Here's how the part is built. I have some questions about the finished solid (model axes, mm). Face numbers are marked on the shaded views. Coordinates: 2 decimals unless noted, no trailing zeros. Order: outer loops, then holes, each group sorted by start corner. A loop starts at its lowest first (then second) coordinate and runs counter-clockwise, first axis right, second up. Notation, with made-up numbers: (59, -30.75) - (109, -30.75) arc R24 cw to (109, -8.75) - close; hole circle Ø8 at (54.5, 13.25). An arc over 180 degrees is marked (long way). Answer in a Markdown table with one row per item. Add a question column.
Item 1: I want a section at B-B (x = 6.5). Please give me the cut outline in (y, z).
Item 2: If I drill on line 1 along Y through (x, z) = (12, 5.5); line 2 along Y through (x, z) = (10.75, 2.75); line 3 along X through (y, z) = (27, 6.25), over which ranges is the centre line in solid material (lowest first)? Write a range as from..to.
Item 3: I want a section at A-A (y = 13.5). Please give me the cut outline in (x, z), plus the area to 3 significant figures.
Item 4: I want a section at C-C (z = 5.25). Please give me the cut outline in (x, y).
Item 5: I want a section at D-D (x = 12). Please give me the cut outline in (y, z).
Item 6: Thinking about a two-plate mould opening in Y: for the marked faces 1, 2, 3 and 4, which applies, +Y half, -Y half, draft (parallel to the pull), parting line (faces both ways), or undercut?
Item 7: Will this pin go through, and if not, where does the flat tip stop? pin 1 Ø11.5 at (x, y) = (12, 17.5) entering from -Z.
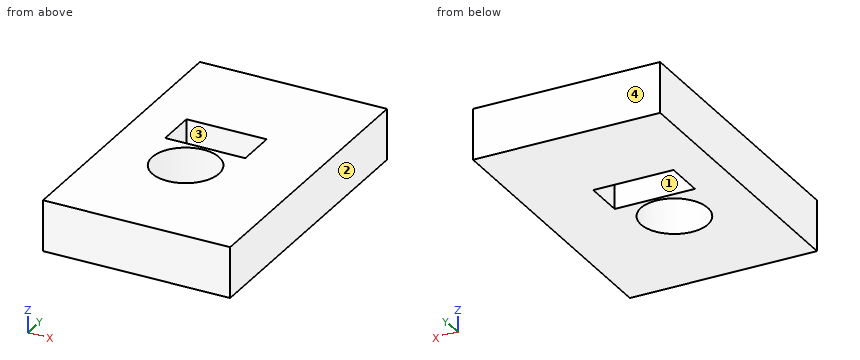
```python
from build123d import *

# Parameters (mm, degrees)
F0_W     = 28
F0_H     = 44
F1_DEPTH = 7.6
F2_R     = 5
F2_W     = 12
F2_H     = 6
F3_DEPTH = 7.601


with BuildPart() as f1:
    # F0 (on Top) → F1 (new body)
    with BuildSketch(Plane.XY):
        with Locations((14, 22)):
            Rectangle(F0_W, F0_H)
    extrude(amount=F1_DEPTH)

    # F2 (on face) → F3 (cut, through all)
    with BuildSketch(Plane.XY.offset(7.6)):
        with Locations((12, 17.5)):
            Circle(F2_R)
        with Locations((12, 26)):
            Rectangle(F2_W, F2_H)
    extrude(amount=-F3_DEPTH, mode=Mode.SUBTRACT)


solid = f1.part
```
Values follow:
| question | item | result |
|---|---|---|
| 1 | outline | (0, 0) - (23, 0) - (23, 7.6) - (0, 7.6) - close; (29, 0) - (44, 0) - (44, 7.6) - (29, 7.6) - close |
| 2 | line 1 | y = 0..12.5, 22.5..23, 29..44 |
| 2 | line 2 | y = 0..12.66, 22.34..23, 29..44 |
| 2 | line 3 | x = 0..6, 18..28 |
| 3 | outline | (0, 0) - (9, 0) - (9, 7.6) - (0, 7.6) - close; (15, 0) - (28, 0) - (28, 7.6) - (15, 7.6) - close |
| 3 | area | 167 mm^2 |
| 4 | outline | (0, 0) - (28, 0) - (28, 44) - (0, 44) - close; hole (6, 23) - (18, 23) - (18, 29) - (6, 29) - close; hole circle Ø10 at (12, 17.5) |
| 5 | outline | (0, 0) - (12.5, 0) - (12.5, 7.6) - (0, 7.6) - close; (22.5, 0) - (23, 0) - (23, 7.6) - (22.5, 7.6) - close; (29, 0) - (44, 0) - (44, 7.6) - (29, 7.6) - close |
| 6 | face 1 | undercut |
| 6 | face 2 | draft |
| 6 | face 3 | undercut |
| 6 | face 4 | +Y half |
| 7 | pin 1 | stops at z = 0 |
